Could you check a few things on this model? Use its own coordinates, in mm. Face numbers are marked on the shaded views. A direction names the side the tool comes from. Give positions to 0.01 mm unless a question says otherwise; leave off trailing zeros. Loops run counter-clockwise (first coordinate to the right, second up) from the corner with the lowest first, then second, coordinate; pieces in that order, holes last. Notation, with made-up numbers: (6, 49) - (17, 49) arc R18 ccw to (17, 71) - close; hole circle Ø5 at (6, -24.75). An arc over 180 degrees is marked (long way). One line per item, written item: value. Start each with the question number.
Q1. I want a section at D-D (y = 8). Please give me the cut outline in (x, z), then the cut area to 3 significant figures.
Q2. I want a section at C-C (x = 2.5). Please give me the cut outline in (y, z), then the cut area to 3 significant figures.
Q3. If we mould it in two halves opening along X, with no side actions, what happens to the marked faces 3, 4, 5 and 6? For each: released by +X, released by -X, zero draft, split by the parting line, or undercut.
Q4. If I drill on line 1 (X direction, y = -11, z = 1.5); line 2 (Y direction, x = 8, z = 14); line 3 (X direction, y = -5.5, z = 25.75), over which ranges is the centre line in solid material (lowest first)? Write a range as from..to.
Q5. I'm going to push flat-ended pins straight in: P1, Ø8, axis at x = -27.5, z = 5.5, coming from the -Y side; P2, Ø12, axis at x = -18, y = 8.5, coming from the +Z side; P3, Ø10, axis at x = -38.5, z = 26, coming from the -Y side; P4, Ø5, axis at y = 3, z = 6, coming from the -X side. Where does each tip first touch, or does it pass through?
Q6. I want a section at A-A (y = -12.5). Please give me the cut outline in (x, z), then the cut area to 3 significant figures.
Q7. For the marked faces 1 and 2, which set-ups out of +Z, -Z, +X, -X, +Y, -Y let a thin tool reach every point of the face, with its end or its side?
Q8. I want a section at B-B (z = 13.75). Please give me the cut outline in (x, y), then the cut area to 4 significant figures.
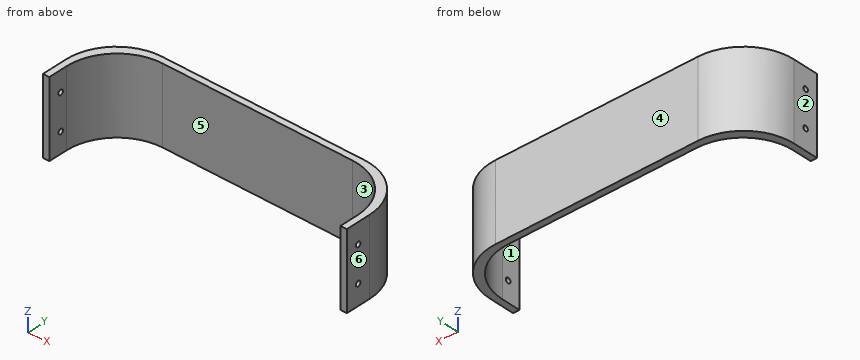
Autodesk Inventor part; units mm, degrees
ref_plane "YZ Plane" through (0, 0, 0) normal (1, 0, 0) x (0, 1, 0)
ref_plane "XZ Plane" through (0, 0, 0) normal (0, 1, 0) x (-1, 0, 0)
ref_plane "XY Plane" through (0, 0, 0) normal (0, 0, 1) x (1, 0, 0)
sketch "Sketch1" plane through (0, 0, 0) normal (0, 0, 1) x (1, 0, 0)
  line L0 (60, 15) -> (-60, 15)
  line L1 (-60, 15) -> (-60, -15)
  line L2 (60, -15) -> (60, 15)
  line L3 (60, 15) -> (-60, -15) construction
  line L4 (-60, 15) -> (60, -15) construction
  line L5 (57.5, 12.5) -> (-57.5, 12.5)
  line L6 (-57.5, 12.5) -> (-57.5, -15)
  line L7 (57.5, -15) -> (57.5, 12.5)
  line L8 (-60, -15) -> (-57.5, -15)
  line L9 (57.5, -15) -> (60, -15)
  point P0 (0, 0)
  dimension "d0" = 120
  dimension "d1" = 30
extrude "Extrusion1" add sketch "Sketch1" along normal blind 30
fillet "Fillet1" radius 20 4 edges at (60, 15, 15) (-60, 15, 15) (-57.5, 12.5, 15) (57.5, 12.5, 15)
sketch "Sketch2" plane through (-60, -15, 0) normal (-1, 0, 0) x (0, 0, 1)
  line L0 (33.379, 5) -> (-9.3676, 5) construction
  line L1 (0, 0) -> (30, 0)
  line L2 (22, 36.2118) -> (22, -4.5967) construction
  line L3 (8, 36.2118) -> (8, -2.8739) construction
  line L4 (30, 10) -> (30, 0) construction
  line L5 (0, 10) -> (0, 0) construction
  circle A0 centre (22, 5) radius 1
  circle A1 centre (8, 5) radius 1
  point P0 (0, 15)
  dimension "d7" = 5
  dimension "d8" = 8
  dimension "d9" = 8
  dimension "d10" = 2
  dimension "d11" = 2
extrude "Extrusion2" cut sketch "Sketch2" against normal blind 120
equation "\"d8\" = d9"
properties part number "Bumper"
Worked answers:
1. outline: (-55.2, 0) - (-50.14, 0) - (-50.14, 30) - (-55.2, 30) - close; (50.14, 0) - (55.2, 0) - (55.2, 30) - (50.14, 30) - close
1. area: 304 mm²
2. outline: (12.5, 0) - (15, 0) - (15, 30) - (12.5, 30) - close
2. area: 75.0 mm²
3. face 3: undercut
3. face 4: zero draft
3. face 5: undercut
3. face 6: released by +X
4. line 1: x = -60..-57.5, 57.5..60
4. line 2: y = 12.5..15
4. line 3: x = -60..-57.4, 57.4..60
5. P1: stops at y = 12.5
5. P2: stops at z = 30
5. P3: stops at y = 11.58
5. P4: stops at x = -59.23
6. outline: (-60, 0) - (-57.5, 0) - (-57.5, 30) - (-60, 30) - close; (57.5, 0) - (60, 0) - (60, 30) - (57.5, 30) - close
6. area: 150 mm²
7. face 1: +Z, -Z, -Y
7. face 2: +Z, -Z, -X, +Y, -Y
8. outline: (-60, -15) - (-57.5, -15) - (-57.5, -7.5) arc R20 cw to (-37.5, 12.5) - (37.5, 12.5) arc R20 cw to (57.5, -7.5) - (57.5, -15) - (60, -15) - (60, -5) arc R20 ccw to (40, 15) - (-40, 15) arc R20 ccw to (-60, -5) - close
8. area: 437.5 mm²
